For this review, take the finished solid that the model builds, in its own axes (mm). Round coordinates to 2 decimals unless told otherwise and drop trailing zeros. Loops run counter-clockwise (first coordinate to the right, second up) from the corner with the lowest first, then second, coordinate; pieces in that order, holes last.
1) Take a section at C-C (x = 113). State the section outline as (y, z) points, then the cut area to 3 significant figures.
2) Take a section at D-D (x = -109.5). State the section outline as (y, z) points.
3) Take a section at A-A (x = 0). State the section outline as (y, z) points, then the cut area to 3 significant figures.
4) Wall thickness on L1, parallel to X at y = -11.5, z = 1; L2, parallel to X at y = -35, z = 3.75; L3, parallel to X at y = -143, z = 1.5: over which ranges is each line inside the solid? List them lowest first.
5) Insertion check: pin 1 (1 mm diameter, centred on x = 92.5, z = 1, fed in from +Y); pin 2 (13 mm diameter, centred on x = 0, y = -140, fed in from +Z); pin 3 (5 mm diameter, centred on x = 140, y = 0, fed in from +Z); pin 4 (1.5 mm diameter, centred on y = 14, z = 6.5, fed in from -X). Each pin has a flat end and moves straight along its axis. Give the tip position at first contact, or say it passes through.
Autodesk Inventor part; units mm, degrees
ref_plane "YZ Plane" through (0, 0, 0) normal (1, 0, 0) x (0, 1, 0)
ref_plane "XZ Plane" through (0, 0, 0) normal (0, 1, 0) x (-1, 0, 0)
ref_plane "XY Plane" through (0, 0, 0) normal (0, 0, 1) x (1, 0, 0)
sketch "Sketch1" plane through (0, 0, 0) normal (0, 0, 1) x (1, 0, 0)
  circle A0 centre (0, 0) radius 105
  circle A1 centre (140, 0) radius 4
  circle A2 centre (140, 0) radius 20
  arc A3 (89.5312, 54.8558) -> (142.8383, 19.7976) centre (153.4821, 94.0385) ccw
  arc A4 (142.8383, -19.7976) -> (89.5312, -54.8558) centre (153.4821, -94.0385) ccw
  circle A5 centre (0, 140) radius 4
  circle A6 centre (0, 140) radius 20
  arc A7 (19.7976, 142.8383) -> (54.8558, 89.5312) centre (94.0385, 153.4821) ccw
  arc A8 (-54.8558, 89.5312) -> (-19.7976, 142.8383) centre (-94.0385, 153.4821) ccw
  circle A9 centre (-140, 0) radius 4
  circle A10 centre (-140, 0) radius 20
  arc A11 (-142.8383, 19.7976) -> (-89.5312, 54.8558) centre (-153.4821, 94.0385) ccw
  arc A12 (-89.5312, -54.8558) -> (-142.8383, -19.7976) centre (-153.4821, -94.0385) ccw
  circle A13 centre (0, -140) radius 4
  circle A14 centre (0, -140) radius 20
  arc A15 (-19.7976, -142.8383) -> (-54.8558, -89.5312) centre (-94.0385, -153.4821) ccw
  arc A16 (54.8558, -89.5313) -> (19.7976, -142.8383) centre (94.0385, -153.4821) ccw
  point P0 (-54.8558, 89.5312)
  point P1 (-89.5312, 54.8558)
  point P2 (-54.8558, -89.5312)
  point P3 (54.8558, -89.5312)
  dimension "d0" = 210
  dimension "d1" = 8
  dimension "d2" = 40
  dimension "d3" = 140
  dimension "d4" = 75
  dimension "d7" = 360
extrude "Extrusion1" add sketch "Sketch1" along normal blind 10
sketch "Sketch2" plane through (0, 0, 0) normal (1, 0, 0) x (0, 1, 0)
  line L0 (-89.5312, 10) -> (-142.8383, 10)
  line L1 (-142.8383, 10) -> (-142.8383, 10)
  line L2 (-142.8383, 10) -> (-89.5312, 10)
  line L3 (-89.5312, 10) -> (-54.8558, 10)
  line L4 (-54.8558, 10) -> (-19.7976, 10)
  line L5 (-19.7976, 10) -> (19.7976, 10)
  line L6 (19.7976, 10) -> (54.8558, 10)
  line L7 (54.8558, 10) -> (89.5312, 10)
  line L8 (89.5312, 10) -> (142.8383, 10)
  line L9 (142.8383, 10) -> (142.8383, 10)
  line L10 (142.8383, 10) -> (89.5312, 10)
  line L11 (89.5312, 10) -> (54.8558, 10)
  line L12 (54.8558, 10) -> (19.7976, 10)
  line L13 (19.7976, 10) -> (-19.7976, 10)
  line L14 (-19.7976, 10) -> (-54.8558, 10)
  line L15 (-54.8558, 10) -> (-89.5312, 10)
  line L16 (-4, 10) -> (4, 10)
  line L17 (136, 10) -> (144, 10)
  line L18 (-4, 10) -> (4, 10)
  line L19 (-144, 10) -> (-136, 10)
  line L20 (-89.5312, 0) -> (-142.8383, 0)
  line L21 (-54.8558, 0) -> (-89.5312, 0)
  line L22 (-19.7976, 0) -> (-54.8558, 0)
  line L23 (19.7976, 0) -> (-19.7976, 0)
  line L24 (54.8558, 0) -> (19.7976, 0)
  line L25 (89.5312, 0) -> (54.8558, 0)
  line L26 (142.8383, 0) -> (89.5312, 0)
  line L27 (142.8383, 0) -> (142.8383, 0)
  line L28 (89.5312, 0) -> (142.8383, 0)
  line L29 (54.8558, 0) -> (89.5312, 0)
  line L30 (19.7976, 0) -> (54.8558, 0)
  line L31 (-19.7976, 0) -> (19.7976, 0)
  line L32 (-54.8558, 0) -> (-19.7976, 0)
  line L33 (-89.5312, 0) -> (-54.8558, 0)
  line L34 (-142.8383, 0) -> (-89.5312, 0)
  line L35 (-142.8383, 0) -> (-142.8383, 0)
  line L36 (-4, 0) -> (4, 0)
  line L37 (136, 0) -> (144, 0)
  line L38 (-4, 0) -> (4, 0)
  line L39 (-144, 0) -> (-136, 0)
  circle A0 centre (-95, -1) radius 7.5
  line L40 (0, 0) -> (0, 10)
  dimension "d11" = 15
  dimension "d12" = 1
  dimension "d13" = 95
revolve "Revolution1" cut sketch "Sketch2" angle 360 about axis through (0, 0, 0) along (0, 0, 1)
properties part number "onderkant base" material "Aluminum 6061"
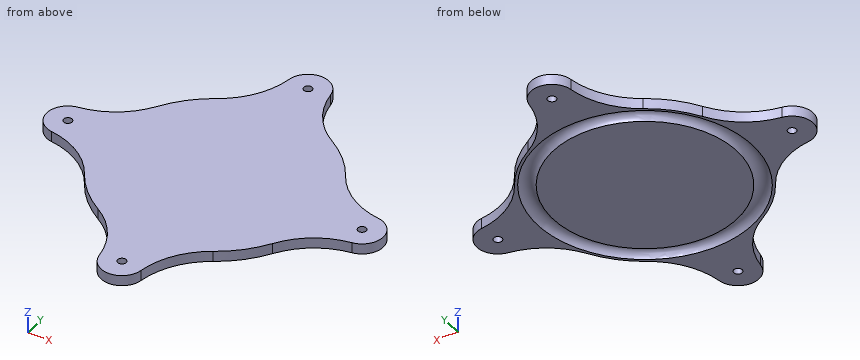
Response:
1. outline: (-30.9, 0) - (30.9, 0) - (30.9, 10) - (-30.9, 10) - close
1. area: 618 mm2
2. outline: (-33.29, 0) - (33.29, 0) - (33.29, 10) - (-33.29, 10) - close
3. outline: (-160, 0) - (-144, 0) - (-144, 10) - (-160, 10) - close; (-136, 0) - (-102.43, 0) arc R7.5 cw to (-87.57, 0) - (87.57, 0) arc R7.5 cw to (102.43, 0) - (136, 0) - (136, 10) - (-136, 10) - close; (144, 0) - (160, 0) - (160, 10) - (144, 10) - close
3. area: 2,890 mm2
4. L1: x = -156.36 to -101.58, -87.01 to 87.01, 101.58 to 156.36
4. L2: x = -107.23 to -94.53, -82.04 to 82.04, 94.53 to 107.23
4. L3: x = -19.77 to -2.65, 2.65 to 19.77
5. pin 1: stops at y = 51.09
5. pin 2: stops at z = 10
5. pin 3: passes through
5. pin 4: stops at x = -154.98
